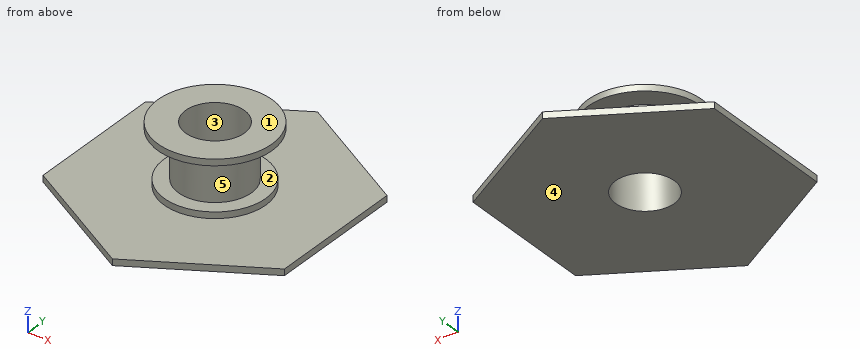
```python
from build123d import *

# Parameters (mm, degrees)
HEX_BASE_DEPTH      = 6.35
SKETCH2_R           = 29.36875
ID_2_DEPTH          = 185.405282824
PIPE_START          = 53.975
SKETCH3_R           = 36.5125
SKETCH3_R_2         = 29.36875
PIPE_DEPTH          = 53.975
FLANGE_START        = 6.35
SKETCH4_R           = 57.15
SKETCH4_R_2         = 29.36875
FLANGE_DEPTH        = 6.35
REINFORCEMENT_START = 6.35
SKETCH5_R           = 50.8
SKETCH5_R_2         = 36.5125
REINFORCEMENT_DEPTH = 6.35


with BuildPart() as part:
    # Sketch1 → hex_base (new body)
    with BuildSketch(Plane.XY):
        Polygon((120.65, 69.657309978), (0, 139.314619955), (-120.65, 69.657309978), (-120.65, -69.657309978), (0, -139.314619955), (120.65, -69.657309978), align=None)
    extrude(amount=HEX_BASE_DEPTH)

    # Sketch2 → ID 2 (cut, through all)
    with BuildSketch(Plane.XY.offset(6.35)):
        Circle(SKETCH2_R)
    extrude(amount=-ID_2_DEPTH, mode=Mode.SUBTRACT)

    # Sketch3 → pipe (add)
    with BuildSketch(Plane.XY.offset(6.35).offset(PIPE_START)):
        Circle(SKETCH3_R)
        Circle(SKETCH3_R_2, mode=Mode.SUBTRACT)
    extrude(amount=-PIPE_DEPTH)

    # Sketch4 → flange (add)
    with BuildSketch(Plane.XY.offset(60.325).offset(FLANGE_START)):
        Circle(SKETCH4_R)
        Circle(SKETCH4_R_2, mode=Mode.SUBTRACT)
    extrude(amount=-FLANGE_DEPTH)

    # Sketch5 → reinforcement (add)
    with BuildSketch(Plane.XY.offset(6.35).offset(REINFORCEMENT_START)):
        Circle(SKETCH5_R)
        Circle(SKETCH5_R_2, mode=Mode.SUBTRACT)
    extrude(amount=-REINFORCEMENT_DEPTH)


solid = part.part
```
The model under review builds one solid part; all positions refer to its coordinate system, in mm. Face numbers are marked on the shaded views. A direction names the side the tool comes from. Round coordinates to 2 decimals unless told otherwise and drop trailing zeros. Write each loop counter-clockwise with the first axis right and the second up, starting at its lowest first coordinate (ties: lowest second). Pieces come first, ordered by that corner, then holes.
(1) We need section B-B on x = 22. Give the boundary of the cut face in (y, z) (3 decimals), and give its area (3 significant figures).
(2) Insertion check: pin 1 (6 mm diameter, centred on x = 21, z = 42.5, fed in from -Y); pin 2 (8 mm diameter, centred on x = -28, z = 13.5, fed in from -Y). Each pin has a flat end and moves straight along its axis. Give the tip position at first contact, or say it passes through.
(3) We need section C-C on z = 39.5. Give the boundary of the cut face in (x, y) (1 decimal).
(4) Mouldability with a two-part tool opening along Y and no side actions: class the marked faces 3, 4 and 5 as +Y half, -Y half, draft (parallel to the pull), parting line (faces both ways), or undercut.
(5) We need section D-D on x = 85.5. Give the boundary of the cut face in (y, z).
(6) Machinability: for the marked faces 1 and 2, which of the approach directions +Z, -Z, +X, -X, +Y, -Y give a long, thin tool a straight path to every point of the face, cutting with its end or side? Answer none if there is none.
(7) Wall thickness on L1, parallel to Y at x = 0, z = 45.5; L2, parallel to X at y = -1, z = 4; L3, parallel to Z at x = -63, y = -73: over which ranges is each line inside the solid? List them lowest first.
Findings below:
1. outline: (-126.613, 0) - (-19.456, 0) - (-19.456, 66.675) - (-52.746, 66.675) - (-52.746, 60.325) - (-29.14, 60.325) - (-29.14, 12.7) - (-45.789, 12.7) - (-45.789, 6.35) - (-126.613, 6.35) - close; (19.456, 0) - (126.613, 0) - (126.613, 6.35) - (45.789, 6.35) - (45.789, 12.7) - (29.14, 12.7) - (29.14, 60.325) - (52.746, 60.325) - (52.746, 66.675) - (19.456, 66.675) - close
1. area: 3,040 mm2
2. pin 1: stops at y = -31.77
2. pin 2: stops at y = -44.73
3. outline: circle Ø73 at (0, 0); hole circle Ø58.7 at (0, 0)
4. face 3: undercut
4. face 4: draft
4. face 5: parting line
5. outline: (-89.95, 0) - (89.95, 0) - (89.95, 6.35) - (-89.95, 6.35) - close
6. face 1: +Z, +X, -X, +Y, -Y
6. face 2: none
7. L1: y = -36.51 to -29.37, 29.37 to 36.51
7. L2: x = -120.65 to -29.35, 29.35 to 120.65
7. L3: z = 0 to 6.35
